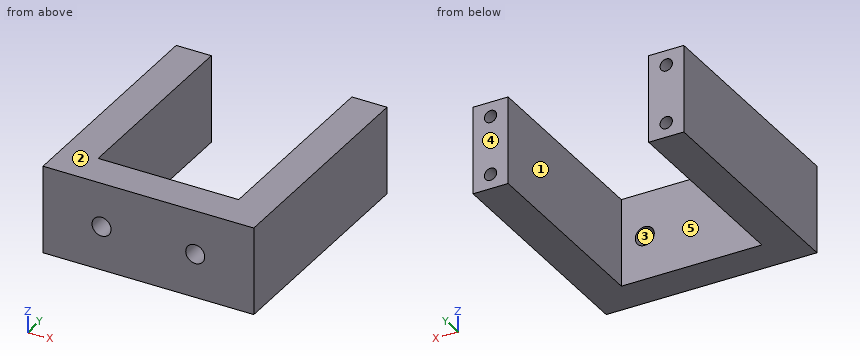
from build123d import *

# Parameters (mm, degrees)
EXTRUDE_1_DEPTH     = 15
M5X0_8_1_D          = 4.2
M5X0_8_1_DEPTH      = 12.4
M5X0_8_1_TIP        = 1.2618073
SKETCH_4_R          = 3.25
CUT_EXTRUDE_1_DEPTH = 79.390050389


with BuildPart() as part:
    # 草图1 → 凸台-拉伸1 (new, symmetric)
    with BuildSketch(Plane.XY):
        Polygon((-36, 80), (-36, 0), (36, 0), (36, 80), (24, 80), (24, 12), (-24, 12), (-24, 80), align=None)
    extrude(amount=EXTRUDE_1_DEPTH, both=True)

    # M5x0.8 螺纹孔1
    with Locations(Plane(origin=(0, 80, 0), x_dir=(-1, 0, 0), z_dir=(0, 1, 0))):
        with Locations((-30, -10), (30, -10), (30, 10), (-30, 10)):
            Hole(M5X0_8_1_D / 2, depth=M5X0_8_1_DEPTH)
            with Locations((0, 0, -(M5X0_8_1_DEPTH + M5X0_8_1_TIP / 2))):  # 118° drill point
                Cone(0, M5X0_8_1_D / 2, M5X0_8_1_TIP, mode=Mode.SUBTRACT)

    # 草图4 → 切除-拉伸1 (cut, through all)
    with BuildSketch(Plane(origin=(0, 12, 0), x_dir=(1, 0, 0), z_dir=(0, 1, 0))):
        with Locations(Location((-16, 0, 0), (0, 0, 270))):
            Circle(SKETCH_4_R)
        with Locations(Location((16, 0, 0), (0, 0, 270))):
            Circle(SKETCH_4_R)
    extrude(amount=-CUT_EXTRUDE_1_DEPTH, mode=Mode.SUBTRACT)


solid = part.part
Check sheet for the modelled part. Datum: model origin and axes. Units: mm. Face numbers are marked on the shaded views. A direction names the side the tool comes from. Round coordinates to 2 decimals unless told otherwise and drop trailing zeros. Order: outer loops, then holes, each group sorted by start corner. A loop starts at its lowest first (then second) coordinate and runs counter-clockwise, first axis right, second up.
Q1. Cross-section at A-A, the plane y = 63. Enter the section's corners in (x, z), plus the area to 3 significant figures.
Filled sheet:
outline: (-36, -15) - (-24, -15) - (-24, 15) - (-36, 15) - close; (24, -15) - (36, -15) - (36, 15) - (24, 15) - close
area: 720 mm2
Q2. Scan lines: L1, parallel to Z at x = 30, y = 74; L2, parallel to X at y = 71.5, z = -10; L3, parallel to X at y = 8.5, z = 0. Record each from-to range of solid material in increasing order.
Filled sheet:
L1: z = -15 to -12.1, -7.9 to 7.9, 12.1 to 15
L2: x = -36 to -32.1, -27.9 to -24, 24 to 27.9, 32.1 to 36
L3: x = -36 to -19.25, -12.75 to 12.75, 19.25 to 36
Q3. Depth check by flat-ended pin: P1, Ø15, axis at x = -8, z = -0.5, coming from the +Y side; P2, Ø1.5, axis at x = -18, z = -9.5, coming from the -Y side; P3, Ø3.5, axis at x = 30, z = 10, coming from the +Y side. Enter the tip coordinate at first touch or a pass-through.
Filled sheet:
P1: stops at y = 12
P2: stops at y = 0
P3: stops at y = 67.39
Q4. Cross-section at D-D, the plane x = -7. Enter the section's corners in (y, z), plus the area to 3 significant figures.
Filled sheet:
outline: (0, -15) - (12, -15) - (12, 15) - (0, 15) - close
area: 360 mm2
Q5. Cross-section at C-C, the plane z = 0. Enter the section's corners in (x, y), plus the area to 3 significant figures.
Filled sheet:
outline: (-36, 0) - (-19.25, 0) - (-19.25, 12) - (-24, 12) - (-24, 80) - (-36, 80) - close; (-12.75, 0) - (12.75, 0) - (12.75, 12) - (-12.75, 12) - close; (19.25, 0) - (36, 0) - (36, 80) - (24, 80) - (24, 12) - (19.25, 12) - close
area: 2,340 mm2
Q6. Draft check along Z on the marked faces 1, 2 and 3. Enter one of: pulls with the +Z half, pulls with the -Z half, needs draft (parallel to the pull), parting line crosses it, or undercut.
Filled sheet:
face 1: needs draft
face 2: pulls with the +Z half
face 3: undercut
Q7. Cross-section at B-B, the plane x = 16. Enter the section's corners in (y, z), plus the area to 3 significant figures.
Filled sheet:
outline: (0, -15) - (12, -15) - (12, -3.25) - (0, -3.25) - close; (0, 3.25) - (12, 3.25) - (12, 15) - (0, 15) - close
area: 282 mm2
Q8. Set-up check for the marked faces 4 and 5: record each of +Z, -Z, +X, -X, +Y, -Y from which the full face is reachable in a straight line by a thin tool's end or side.
Filled sheet:
face 4: +Z, -Z, +X, -X, +Y
face 5: +Z, -Z, +Y
